```python
from build123d import *

# Parameters (mm, degrees)
EXTRUDE_1_DEPTH     = 25
SKETCH_2_R          = 2
CUT_EXTRUDE_1_DEPTH = 35.263683398
SKETCH_3_R          = 3
CUT_EXTRUDE_2_DEPTH = 31.987900865
CHAMFER_1_SIZE      = 0.5


with BuildPart() as part:
    # 스케치1 → 보스-돌출1 (new body)
    with BuildSketch(Plane.XY):
        Polygon((-15, -7.5), (-10, -7.5), (-4.803847577, -10.5), (4.803847577, -10.5), (10, -7.5), (15, -7.5), (15, 7.5), (-15, 7.5), align=None)
    extrude(amount=EXTRUDE_1_DEPTH)

    # 스케치2 → 컷-돌출1 (cut, through all)
    with BuildSketch(Plane(origin=(0, 7.5, 0), x_dir=(1, 0, 0), z_dir=(0, 1, 0))):
        with Locations(Location((-10, -5, 0), (0, 0, 270))):
            Circle(SKETCH_2_R)
        with Locations(Location((-10, -20, 0), (0, 0, 270))):
            Circle(SKETCH_2_R)
        with Locations(Location((10, -20, 0), (0, 0, 270))):
            Circle(SKETCH_2_R)
        with Locations(Location((10, -5, 0), (0, 0, 270))):
            Circle(SKETCH_2_R)
    extrude(amount=-CUT_EXTRUDE_1_DEPTH, mode=Mode.SUBTRACT)

    # 스케치3 → 컷-돌출2 (cut, through all)
    with BuildSketch(Plane.XY.offset(25)):
        with Locations((0, -1.5)):
            Circle(SKETCH_3_R)
    extrude(amount=-CUT_EXTRUDE_2_DEPTH, mode=Mode.SUBTRACT)

    # 모따기1
    chamfer_1_edges = [part.edges().sort_by_distance(p)[0] for p in [
        (0, 7.5, 0),
        (-15, 7.5, 12.5),
        (15, 7.5, 12.5),
        (-10, 7.5, 3),
        (-10, 7.5, 18),
        (10, 7.5, 18),
        (10, 7.5, 3),
        (0, 7.5, 25),
    ]]
    chamfer(chamfer_1_edges, length=CHAMFER_1_SIZE)


solid = part.part
```
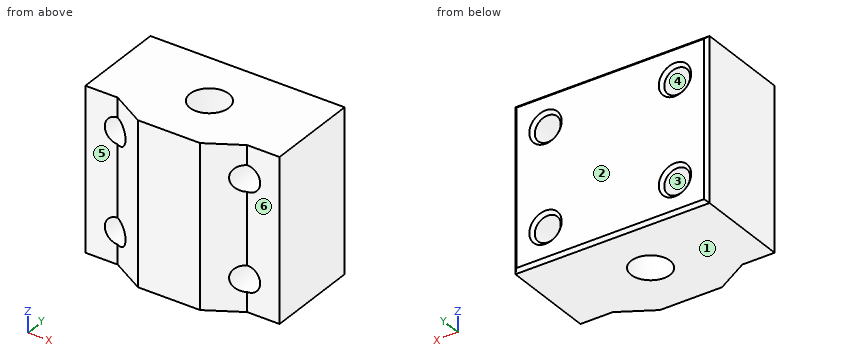
The model under review builds one solid part; all positions refer to its coordinate system, in mm. Face numbers are marked on the shaded views. A direction names the side the tool comes from. Round coordinates to 2 decimals unless told otherwise and drop trailing zeros. Order: outer loops, then holes, each group sorted by start corner. A loop starts at its lowest first (then second) coordinate and runs counter-clockwise, first axis right, second up.
(1) Take a section at D-D, the plane x = 0. State the section outline as (y, z) points.
Working result:
outline: (-10.5, 0) - (-4.5, 0) - (-4.5, 25) - (-10.5, 25) - close; (1.5, 0) - (7, 0) - (7.5, 0.5) - (7.5, 24.5) - (7, 25) - (1.5, 25) - close
(2) For P1, Ø6.5, axis at x = 10, z = 20, coming from the -Y side; P2, Ø5, axis at x = -8.5, z = 20, coming from the -Y side; P3, Ø1.5, axis at x = -12.5, z = 14, coming from the -Y side, all flat-tipped, find the tip position at first contact; note any pin that passes through.
Working result:
P1: stops at y = -9.38
P2: stops at y = -9.81
P3: stops at y = -7.5
(3) Tool access review of the marked faces 4, 5 and 6: name each direction out of +Z, -Z, +X, -X, +Y, -Y from which nothing blocks a thin tool from reaching the whole face with its end or side.
Working result:
face 4: +Y, -Y
face 5: +Z, -Z, -X, -Y
face 6: +Z, -Z, +X, -Y
(4) Wall thickness on L1, parallel to Z at x = -10, y = 1.5; L2, parallel to Y at x = 0, z = 12; L3, parallel to X at y = 0.75, z = 20: over which ranges is each line inside the solid? List them lowest first.
Working result:
L1: z = 0 to 3, 7 to 18, 22 to 25
L2: y = -10.5 to -4.5, 1.5 to 7.5
L3: x = -15 to -12, -8 to -1.98, 1.98 to 8, 12 to 15
(5) Take a section at C-C, the plane y = 3. State the section outline as (x, z) points.
Working result:
outline: (-15, 0) - (15, 0) - (15, 25) - (-15, 25) - close; hole circle Ø4 at (-10, 5); hole circle Ø4 at (-10, 20); hole circle Ø4 at (10, 5); hole circle Ø4 at (10, 20)
(6) Mouldability with a two-part tool opening along Z and no side actions: class the marked faces 1, 2 and 3 as released by +Z, released by -Z, zero draft, split by the parting line, or undercut.
Working result:
face 1: released by -Z
face 2: zero draft
face 3: undercut
(7) Take a section at A-A, the plane y = -1.5. State the section outline as (x, z) points, plus the area to 3 significant figures.
Working result:
outline: (-15, 0) - (-3, 0) - (-3, 25) - (-15, 25) - close; (3, 0) - (15, 0) - (15, 25) - (3, 25) - close; hole circle Ø4 at (-10, 5); hole circle Ø4 at (-10, 20); hole circle Ø4 at (10, 5); hole circle Ø4 at (10, 20)
area: 550 mm2
(8) Take a section at B-B, the plane z = 5. State the section outline as (x, y) points.
Working result:
outline: (-15, -7.5) - (-12, -7.5) - (-12, 7) - (-12.5, 7.5) - (-14.5, 7.5) - (-15, 7) - close; (-8, -8.65) - (-4.8, -10.5) - (4.8, -10.5) - (8, -8.65) - (8, 7) - (7.5, 7.5) - (-7.5, 7.5) - (-8, 7) - close; (12, -7.5) - (15, -7.5) - (15, 7) - (14.5, 7.5) - (12.5, 7.5) - (12, 7) - close; hole circle Ø6 at (0, -1.5)
